```python
from build123d import *

# Parameters (mm, degrees)
F0_W     = 2
F0_H     = 30
F1_DEPTH = 26
F2_R     = 5
F3_DEPTH = 40.2
F4_R     = 5
F5_DEPTH = 23
F6_R     = 5


with BuildPart() as f1:
    # F0 (on Right) → F1 (new body)
    with BuildSketch(Plane.YZ):
        Rectangle(F0_W, F0_H)
        Polygon((1, -15), (-1, -15), (-1, -17), (35, -17), (35, -15), (33, -15), align=None)
        with Locations((34, 0)):
            Rectangle(F0_W, F0_H)
    extrude(amount=F1_DEPTH)

    # F2 (on Front) → F3 (cut)
    with BuildSketch(Plane.XZ):
        with Locations((13, 0)):
            Circle(F2_R)
    extrude(amount=-F3_DEPTH, mode=Mode.SUBTRACT)

    # F4 (on Front) → F5 (cut)
    with BuildSketch(Plane.XZ):
        with Locations((13, 0)):
            Circle(F4_R)
    extrude(amount=F5_DEPTH, mode=Mode.SUBTRACT)

    # F6
    f6_edges = [f1.edges().sort_by_distance(p)[0] for p in [
        (26, 0, 15),
        (26, 34, 15),
        (0, 0, 15),
        (0, 34, 15),
    ]]
    fillet(f6_edges, radius=F6_R)


solid = f1.part
```
Geometry check sheet. Reference: the model listing, model coordinates, mm. A direction names the side the tool comes from. Round coordinates to 2 decimals unless told otherwise and drop trailing zeros. Loops run counter-clockwise (first coordinate to the right, second up) from the corner with the lowest first, then second, coordinate; pieces in that order, holes last. Notation, with made-up numbers: M 77.25,81.5 L 124.25,81.5 A10 ccw 124.25,100.5 Z; hole C 43,-35 d9. An arc over 180 degrees is marked long. Return JSON: item names as keys, results as strings. Group by question number.
(1) Set-up check for faces 1 (the face through (13, 17, -17)), 2 (the face through (13, 17, -15)): record each of +Z, -Z, +X, -X, +Y, -Y from which the full face is reachable in a straight line by a thin tool's end or side.
(2) Section check D-D, the plane z = 4.5. Enter the section's corners in (x, y), and give its area (3 significant figures).
(3) Go/stop test with a flat-tipped pin: pin 1 (6 mm diameter, centred on x = 11.5, y = 29.5, fed in from +Z). Record where the tip stops, or that it passes through.
(4) Section check B-B, the plane x = 13. Enter the section's corners in (y, z).
(5) Section check C-C, the plane x = 7. Enter the section's corners in (y, z), and give its area (3 significant figures).
(6) Scan lines: line 1 along Y through (x, z) = (15.5, 6); line 2 along Z through (x, y) = (13, 0.55); line 3 along Z through (x, y) = (4.5, 11). Record each from-to range of solid material in increasing order. Write a range as [from, to].
(7) Section check A-A, the plane z = -11.5. Enter the section's corners in (x, y), and give its area (3 significant figures).
(8) Mould release check, pull along Y, two halves, no side actions. Record for faces 3 (the face through (24, 0, 14)), 4 (the face through (7, 1, 0)), 5 (the face through (9.9, -1, -4.3)), 6 (the face through (7, 33, 0)): pulls with the +Y half, pulls with the -Y half, needs draft (parallel to the pull), parting line crosses it, or undercut.
Data:
{
 "1": {"face 1": "-Z, +X, -X, +Y, -Y", "face 2": "+Z, +X, -X"},
 "2": {"outline": "M 0,-1 L 10.82,-1 L 10.82,1 L 0,1 Z; M 0,33 L 10.82,33 L 10.82,35 L 0,35 Z; M 15.18,-1 L 26,-1 L 26,1 L 15.18,1 Z; M 15.18,33 L 26,33 L 26,35 L 15.18,35 Z", "area": "86.6 mm²"},
 "3": {"pin 1": "z = -15"},
 "4": {"outline": "M -1,-17 L 35,-17 L 35,-5 L 33,-5 L 33,-15 L 1,-15 L 1,-5 L -1,-5 Z; M -1,5 L 1,5 L 1,15 L -1,15 Z; M 33,5 L 35,5 L 35,15 L 33,15 Z"},
 "5": {"outline": "M -1,-17 L 35,-17 L 35,15 L 33,15 L 33,-15 L 1,-15 L 1,15 L -1,15 Z", "area": "192 mm²"},
 "6": {"line 1": "[-1, 1], [33, 35]", "line 2": "[-17, -5], [5, 15]", "line 3": "[-17, -15]"},
 "7": {"outline": "M 0,-1 L 26,-1 L 26,1 L 0,1 Z; M 0,33 L 26,33 L 26,35 L 0,35 Z", "area": "104 mm²"},
 "8": {"face 3": "needs draft", "face 4": "undercut", "face 5": "pulls with the -Y half", "face 6": "undercut"}
}
